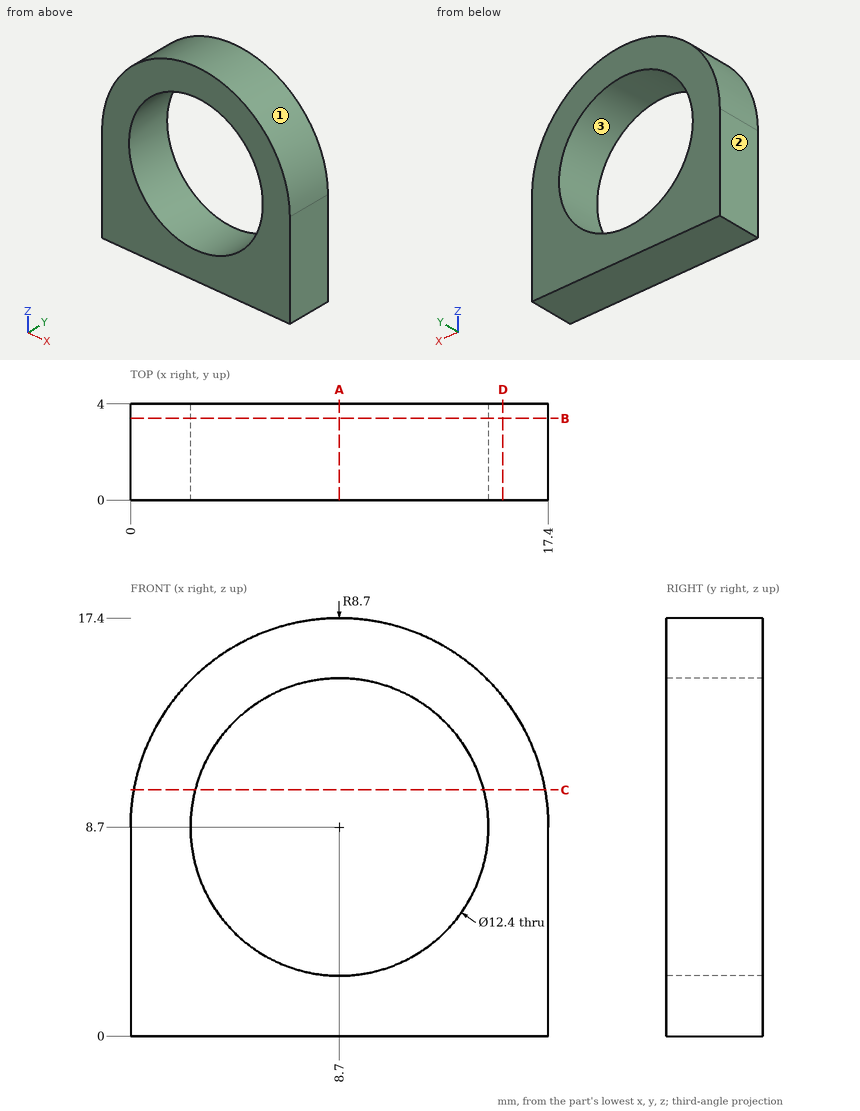
Verification items for this drawing (mm, ordinates from the low corner). Coordinates: 2 decimals unless noted, no trailing zeros. Write each loop counter-clockwise with the first axis right and the second up, starting at its lowest first coordinate (ties: lowest second). Pieces come first, ordered by that corner, then holes. Notation, with made-up numbers: M -6.5,-38.75 L 11.5,-38.75 A26 cw 11.5,-21.75 Z; hole C 40,45.5 d11. An arc over 180 degrees is marked long. Answer as a JSON object with one key per item and string values. Group by question number.
(1) Material ranges on line 1 (Z direction, x = 8.7, y = 2.6); line 2 (X direction, y = 3.15, z = 5.75), recorded low to high.
(2) Release check for a two-part mould opening along Z. For the marked faces 1, 2 and 3 record: +Z half, -Z half, draft (parallel to the pull), parting line (faces both ways), or undercut.
(3) Cross-section at B-B, the plane y = 3.4. Record the cut outline in (x, z), and give its area (3 significant figures).
(4) Cross-section at D-D, the plane x = 15.5. Record the cut outline in (y, z).
(5) Gauge pin test, flat end, axial feed: pin 1 (7.5 mm diameter, centred on x = 8.7, z = 8.7, fed in from -Y). Record the tip position at first contact, or that the pin passes through.
(6) Cross-section at C-C, the plane z = 10.25. Record the cut outline in (x, y), and give its area (3 significant figures).
(7) Cross-section at A-A, the plane x = 8.7. Record the cut outline in (y, z), and give its area (3 significant figures).
Reply:
{
 "1": {"line 1": "0 to 2.5, 14.9 to 17.4", "line 2": "0 to 3.25, 14.15 to 17.4"},
 "2": {"face 1": "+Z half", "face 2": "draft", "face 3": "undercut"},
 "3": {"outline": "M 0,0 L 17.4,0 L 17.4,8.7 A8.7 ccw 0,8.7 Z; hole C 8.7,8.7 d12.4", "area": "150 mm²"},
 "4": {"outline": "M 0,0 L 4,0 L 4,14.13 L 0,14.13 Z"},
 "5": {"pin 1": "through"},
 "6": {"outline": "M 0.14,0 L 2.7,0 L 2.7,4 L 0.14,4 Z; M 14.7,0 L 17.26,0 L 17.26,4 L 14.7,4 Z", "area": "20.5 mm²"},
 "7": {"outline": "M 0,0 L 4,0 L 4,2.5 L 0,2.5 Z; M 0,14.9 L 4,14.9 L 4,17.4 L 0,17.4 Z", "area": "20.0 mm²"}
}
